```python
from build123d import *

# Parameters (mm, degrees)
SKETCH1_W           = 88.9
SKETCH1_H           = 12.7
SKETCH1_R           = 2.54
BOSS_EXTRUDE2_DEPTH = 5.08
SKETCH3_R           = 4.7625
CUT_EXTRUDE1_DEPTH  = 2.54
SKETCH4_W           = 31.75
SKETCH4_H           = 31.75
SKETCH4_R           = 6.985
BOSS_EXTRUDE3_DEPTH = 12.7
FILLET1_R           = 2.54


with BuildPart() as part:
    # Sketch1 → Boss-Extrude2 (new body)
    with BuildSketch(Plane(origin=(0, 0, 0), x_dir=(1, 0, 0), z_dir=(0, 1, 0))):
        with Locations((44.45, 6.35)):
            Rectangle(SKETCH1_W, SKETCH1_H)
        with Locations(Location((6.35, 6.35, 0), (0, 0, 270))):
            Circle(SKETCH1_R, mode=Mode.SUBTRACT)
        with Locations(Location((82.55, 6.35, 0), (0, 0, 270))):
            Circle(SKETCH1_R, mode=Mode.SUBTRACT)
    extrude(amount=BOSS_EXTRUDE2_DEPTH)

    # Sketch3 → Cut-Extrude1 (cut)
    with BuildSketch(Plane(origin=(0, 5.08, 0), x_dir=(1, 0, 0), z_dir=(0, 1, 0))):
        with Locations(Location((6.35, 6.35, 0), (0, 0, 270))):
            Circle(SKETCH3_R)
        with Locations(Location((82.55, 6.35, 0), (0, 0, 270))):
            Circle(SKETCH3_R)
    extrude(amount=-CUT_EXTRUDE1_DEPTH, mode=Mode.SUBTRACT)

    # Sketch4 → Boss-Extrude3 (add)
    with BuildSketch(Plane.XY):
        with Locations((44.45, 15.875)):
            Rectangle(SKETCH4_W, SKETCH4_H)
        with Locations((44.45, 16.9545)):
            Circle(SKETCH4_R, mode=Mode.SUBTRACT)
    extrude(amount=-BOSS_EXTRUDE3_DEPTH)

    # Fillet1
    fillet1_edges = [part.edges().sort_by_distance(p)[0] for p in [
        (37.465, 16.9545, -12.7),
        (60.325, 31.75, -6.35),
        (28.575, 5.08, -6.35),
        (28.575, 31.75, -6.35),
        (60.325, 5.08, -6.35),
        (37.465, 16.9545, 0),
    ]]
    fillet(fillet1_edges, radius=FILLET1_R)


solid = part.part
```
Can you work these out from the model? Positions are in its coordinate system, mm. A direction names the side the tool comes from. Round coordinates to 2 decimals unless told otherwise and drop trailing zeros. Loops run counter-clockwise (first coordinate to the right, second up) from the corner with the lowest first, then second, coordinate; pieces in that order, holes last. Notation, with made-up numbers: M -19.5,5.25 L 24.5,5.25 A18 cw 24.5,25.25 Z; hole C 17,3 d4. An arc over 180 degrees is marked long. Answer in a Markdown table with one row per item.
1. If we section it at B-B, the plane z = -6.35: Give the number of separate pieces and of enclosed holes in the cut face, plus the area to 3 significant figures.
Established:
| item | result |
|---|---|
| separate pieces | 3 |
| enclosed holes | 1 |
| area | 1,070 mm² |
2. If we section it at D-D, the plane y = 6.5: Please give me the cut outline in (x, z), plus the area to 3 significant figures.
Established:
| item | result |
|---|---|
| outline | M 28.31,-12.7 L 60.59,-12.7 L 60.59,0 L 28.31,0 Z |
| area | 410 mm² |
3. Please list where these lines run through material, in increasing order: line 1 (X direction, y = 2.5, z = -6.5); line 2 (Z direction, x = 82.55, y = 0.85); line 3 (Y direction, x = 69, z = -9.5). Write a range as from..to.
Established:
| item | result |
|---|---|
| line 1 | 0..3.81, 8.89..80.01, 85.09..88.9 |
| line 2 | -12.7..-8.89, -3.81..0 |
| line 3 | 0..5.08 |
4. I'm going to push flat-ended pins straight in: pin 1 Ø5 at (x, z) = (5, -6.5) entering from +Y; pin 2 Ø2 at (y, z) = (7.5, -9) entering from -X; pin 3 Ø2 at (y, z) = (27.5, -1.5) entering from -X (3 decimals). Where does each tip first touch, or does it pass through?
Established:
| item | result |
|---|---|
| pin 1 | y = 2.54 |
| pin 2 | x = 28.31 |
| pin 3 | x = 28.575 |
5. If we section it at C-C, the plane x = 6.35: Please give me the cut outline in (y, z), plus the area to 3 significant figures.
Established:
| item | result |
|---|---|
| outline | M 0,-12.7 L 5.08,-12.7 L 5.08,-11.11 L 2.54,-11.11 L 2.54,-8.89 L 0,-8.89 Z; M 0,-3.81 L 2.54,-3.81 L 2.54,-1.59 L 5.08,-1.59 L 5.08,0 L 0,0 Z |
| area | 27.4 mm² |
6. On a 3-axis mill with a long thin cutter (end or side, diameter ignored), from which of +Z, -Z, +X, -X, +Y, -Y can I reach the whole of each face in a straight line? I mean faces 1 (the face through (3.45, 3.83, -10.13)), 2 (the face through (73, 5.08, -6)), 3 (the face through (37.47, 17.26, -6.3)), 4 (the face through (28.575, 18, -6)). Say none if no direction works.
Established:
| item | result |
|---|---|
| face 1 | +Y |
| face 2 | +Z, -Z, +X, +Y |
| face 3 | +Z, -Z |
| face 4 | +Z, -Z, -X, +Y |
7. If we section it at A-A, the plane x = 44.45: Please give me the cut outline in (y, z), plus the area to 3 significant figures.
Established:
| item | result |
|---|---|
| outline | M 0,-12.7 L 7.43,-12.7 A2.54 ccw 9.97,-10.16 L 9.97,-2.54 A2.54 ccw 7.43,0 L 0,0 Z; M 23.94,-10.16 A2.54 ccw 26.48,-12.7 L 31.75,-12.7 L 31.75,0 L 26.48,0 A2.54 ccw 23.94,-2.54 Z |
| area | 220 mm² |
8. Thinking about a two-plate mould opening in X: for faces 5 (the face through (44, 0, -6)), 6 (the face through (60.325, 18, -6)), 7 (the face through (8.87, 1.25, -6.68)), which applies, pulls with the +X half, pulls with the -X half, needs draft (parallel to the pull), parting line crosses it, or undercut?
Established:
| item | result |
|---|---|
| face 5 | needs draft |
| face 6 | pulls with the +X half |
| face 7 | undercut |
